Work out the finished part from the listing and answer in its coordinate system (mm). Face numbers are marked on the shaded views. A direction names the side the tool comes from. Round coordinates to 2 decimals unless told otherwise and drop trailing zeros. Loops run counter-clockwise (first coordinate to the right, second up) from the corner with the lowest first, then second, coordinate; pieces in that order, holes last. Notation, with made-up numbers: (-4, 18) - (7, 18) arc R20 cw to (7, 49) - close; hole circle Ø6 at (20.5, 15). An arc over 180 degrees is marked (long way). Answer as CSV lines item,"result". Start each with the question number.
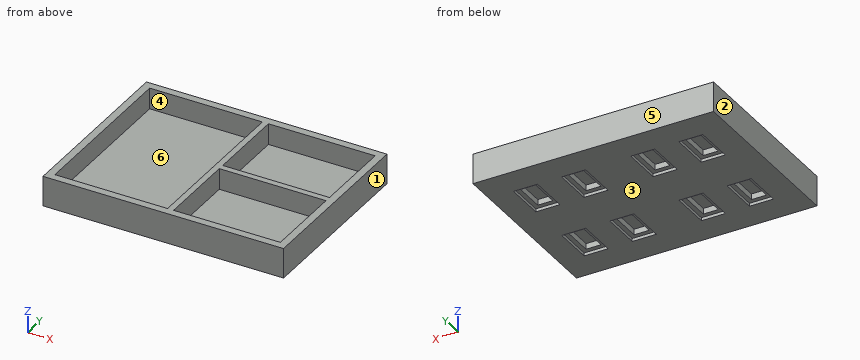
```python
from build123d import *

# Parameters (mm, degrees)
F0_W     = 35.5
F0_H     = 26.5
F1_DEPTH = 10
F0_W_2   = 37.5
F0_H_2   = 27.5
F0_W_3   = 8.0000035167
F0_H_3   = 13.0000035167
F0_W_4   = 8
F0_H_4   = 13
F0_W_5   = 5
F0_H_5   = 10
F2_DEPTH = 3
F3_DEPTH = 1
F4_DEPTH = 2.9


with BuildPart() as f1:
    # F0 (on Top) → F1 (new body)
    with BuildSketch(Plane.XY):
        Polygon((0, 30), (0, 0), (80, 0), (80, 60), (0, 60), align=None)
        with Locations((59.75, 15.75)):
            Rectangle(F0_W, F0_H, mode=Mode.SUBTRACT)
        Polygon((2.5, 57.5), (40, 57.5), (40, 30), (40, 2.5), (2.5, 2.5), (2.5, 30), align=None, mode=Mode.SUBTRACT)
        with Locations((59.75, 44.25)):
            Rectangle(F0_W, F0_H, mode=Mode.SUBTRACT)
    extrude(amount=F1_DEPTH)

    # F0 (on Top) → F2 (join)
    with BuildSketch(Plane.XY):
        with Locations((21.25, 43.75)):
            Rectangle(F0_W_2, F0_H_2)
        with Locations((13, 44)):
            Rectangle(F0_W_3, F0_H_3, mode=Mode.SUBTRACT)
        with Locations((29, 44)):
            Rectangle(F0_W_3, F0_H_3, mode=Mode.SUBTRACT)
        with Locations((21.25, 16.25)):
            Rectangle(F0_W_2, F0_H_2)
        with Locations((13, 16)):
            Rectangle(F0_W_3, F0_H_3, mode=Mode.SUBTRACT)
        with Locations((29, 16)):
            Rectangle(F0_W_3, F0_H_3, mode=Mode.SUBTRACT)
        with Locations((59.75, 44.25)):
            Rectangle(F0_W, F0_H)
        with Locations((52, 44)):
            Rectangle(F0_W_4, F0_H_4, mode=Mode.SUBTRACT)
        with Locations((68, 44)):
            Rectangle(F0_W_4, F0_H_4, mode=Mode.SUBTRACT)
        with Locations((59.75, 15.75)):
            Rectangle(F0_W, F0_H)
        with Locations((52, 16)):
            Rectangle(F0_W_4, F0_H_4, mode=Mode.SUBTRACT)
        with Locations((68, 16)):
            Rectangle(F0_W_4, F0_H_4, mode=Mode.SUBTRACT)
        with Locations((13, 44)):
            Rectangle(F0_W_3, F0_H_3)
        with Locations((13, 44)):
            Rectangle(F0_W_5, F0_H_5, mode=Mode.SUBTRACT)
        with Locations((29, 44)):
            Rectangle(F0_W_3, F0_H_3)
        with Locations((29, 44)):
            Rectangle(F0_W_5, F0_H_5, mode=Mode.SUBTRACT)
        with Locations((29, 16)):
            Rectangle(F0_W_3, F0_H_3)
        with Locations((29, 16)):
            Rectangle(F0_W_5, F0_H_5, mode=Mode.SUBTRACT)
        with Locations((13, 16)):
            Rectangle(F0_W_3, F0_H_3)
        with Locations((13, 16)):
            Rectangle(F0_W_5, F0_H_5, mode=Mode.SUBTRACT)
        with Locations((52, 44)):
            Rectangle(F0_W_4, F0_H_4)
        with Locations((52, 44)):
            Rectangle(F0_W_5, F0_H_5, mode=Mode.SUBTRACT)
        with Locations((68, 44)):
            Rectangle(F0_W_4, F0_H_4)
        with Locations((68, 44)):
            Rectangle(F0_W_5, F0_H_5, mode=Mode.SUBTRACT)
        with Locations((68, 16)):
            Rectangle(F0_W_4, F0_H_4)
        with Locations((68, 16)):
            Rectangle(F0_W_5, F0_H_5, mode=Mode.SUBTRACT)
        with Locations((52, 16)):
            Rectangle(F0_W_4, F0_H_4)
        with Locations((52, 16)):
            Rectangle(F0_W_5, F0_H_5, mode=Mode.SUBTRACT)
        with Locations((13, 44)):
            Rectangle(F0_W_5, F0_H_5)
        with Locations((29, 44)):
            Rectangle(F0_W_5, F0_H_5)
        with Locations((52, 44)):
            Rectangle(F0_W_5, F0_H_5)
        with Locations((68, 44)):
            Rectangle(F0_W_5, F0_H_5)
        with Locations((68, 16)):
            Rectangle(F0_W_5, F0_H_5)
        with Locations((52, 16)):
            Rectangle(F0_W_5, F0_H_5)
        with Locations((29, 16)):
            Rectangle(F0_W_5, F0_H_5)
        with Locations((13, 16)):
            Rectangle(F0_W_5, F0_H_5)
    extrude(amount=F2_DEPTH)

    # F0 (on Top) → F3 (cut)
    with BuildSketch(Plane.XY):
        with Locations((68, 44)):
            Rectangle(F0_W_4, F0_H_4)
        with Locations((68, 44)):
            Rectangle(F0_W_5, F0_H_5, mode=Mode.SUBTRACT)
        with Locations((52, 44)):
            Rectangle(F0_W_4, F0_H_4)
        with Locations((52, 44)):
            Rectangle(F0_W_5, F0_H_5, mode=Mode.SUBTRACT)
        with Locations((52, 16)):
            Rectangle(F0_W_4, F0_H_4)
        with Locations((52, 16)):
            Rectangle(F0_W_5, F0_H_5, mode=Mode.SUBTRACT)
        with Locations((68, 16)):
            Rectangle(F0_W_4, F0_H_4)
        with Locations((68, 16)):
            Rectangle(F0_W_5, F0_H_5, mode=Mode.SUBTRACT)
        with Locations((29, 44)):
            Rectangle(F0_W_3, F0_H_3)
        with Locations((29, 44)):
            Rectangle(F0_W_5, F0_H_5, mode=Mode.SUBTRACT)
        with Locations((13, 44)):
            Rectangle(F0_W_3, F0_H_3)
        with Locations((13, 44)):
            Rectangle(F0_W_5, F0_H_5, mode=Mode.SUBTRACT)
        with Locations((13, 16)):
            Rectangle(F0_W_3, F0_H_3)
        with Locations((13, 16)):
            Rectangle(F0_W_5, F0_H_5, mode=Mode.SUBTRACT)
        with Locations((29, 16)):
            Rectangle(F0_W_3, F0_H_3)
        with Locations((29, 16)):
            Rectangle(F0_W_5, F0_H_5, mode=Mode.SUBTRACT)
    extrude(amount=F3_DEPTH, mode=Mode.SUBTRACT)

    # F0 (on Top) → F4 (cut)
    with BuildSketch(Plane.XY):
        with Locations((68, 44)):
            Rectangle(F0_W_5, F0_H_5)
        with Locations((52, 44)):
            Rectangle(F0_W_5, F0_H_5)
        with Locations((29, 44)):
            Rectangle(F0_W_5, F0_H_5)
        with Locations((13, 44)):
            Rectangle(F0_W_5, F0_H_5)
        with Locations((13, 16)):
            Rectangle(F0_W_5, F0_H_5)
        with Locations((29, 16)):
            Rectangle(F0_W_5, F0_H_5)
        with Locations((52, 16)):
            Rectangle(F0_W_5, F0_H_5)
        with Locations((68, 16)):
            Rectangle(F0_W_5, F0_H_5)
    extrude(amount=F4_DEPTH, mode=Mode.SUBTRACT)


solid = f1.part
```
Item 1: Flat-ended cylindrical pins translate along their axes: pin 1 Ø4 at (x, y) = (60.5, 16) entering from +Z; pin 2 Ø6.5 at (x, y) = (68.5, 13) entering from -Z. Find the tip coordinate at first contact, or state that the pin passes through.
Item 2: Find the intervals of material crossed by L1, parallel to Y at x = 71, z = 8; L2, parallel to Y at x = 12.5, z = 2.5; L3, parallel to X at y = 38.5, z = 3.75, in increasing order.
Item 3: Section B-B, the plane x = 45 is taken. Give the vertices of the cut face in (y, z).
Item 4: Which of the six approach directions +Z, -Z, +X, -X, +Y, -Y give full straight-line access (tool end or side, diameter ignored) to the marked faces 5 and 6?
Item 5: Section D-D, the plane x = 35.5 is taken. Give the vertices of the cut face in (y, z).
Item 6: Section A-A, the plane z = 4.5 is taken. Give the vertices of the cut face in (x, y), and give its area (3 significant figures).
Item 7: Determine the mould class of the marked faces 1, 2, 3 and 4 for opening direction X: pulls with the +X half, pulls with the -X half, needs draft (parallel to the pull), parting line crosses it, or undercut.
Item 8: Section C-C, the plane y = 54 is taken. Give the vertices of the cut face in (x, z).
Answer:
1,pin 1,"stops at z = 3"
1,pin 2,"stops at z = 1"
2,L1,"y = 0 to 2.5, 29 to 31, 57.5 to 60"
2,L2,"y = 0 to 11, 21 to 39, 49 to 60"
2,L3,"x = 0 to 2.5, 40 to 42, 77.5 to 80"
3,outline,"(0, 0) - (60, 0) - (60, 10) - (57.5, 10) - (57.5, 3) - (31, 3) - (31, 10) - (29, 10) - (29, 3) - (2.5, 3) - (2.5, 10) - (0, 10) - close"
4,face 5,"+Z, -Z, +X, -X, +Y"
4,face 6,"+Z"
5,outline,"(0, 0) - (60, 0) - (60, 10) - (57.5, 10) - (57.5, 3) - (2.5, 3) - (2.5, 10) - (0, 10) - close"
6,outline,"(0, 0) - (80, 0) - (80, 60) - (0, 60) - close; hole (2.5, 2.5) - (40, 2.5) - (40, 57.5) - (2.5, 57.5) - close; hole (42, 2.5) - (77.5, 2.5) - (77.5, 29) - (42, 29) - close; hole (42, 31) - (77.5, 31) - (77.5, 57.5) - (42, 57.5) - close"
6,area,"856 mm²"
7,face 1,"pulls with the +X half"
7,face 2,"pulls with the -X half"
7,face 3,"needs draft"
7,face 4,"undercut"
8,outline,"(0, 0) - (80, 0) - (80, 10) - (77.5, 10) - (77.5, 3) - (42, 3) - (42, 10) - (40, 10) - (40, 3) - (2.5, 3) - (2.5, 10) - (0, 10) - close"
